Build history of the part. All positions in model axes, mm. Round coordinates to 2 decimals unless told otherwise and drop trailing zeros. Write each loop counter-clockwise with the first axis right and the second up, starting at its lowest first coordinate (ties: lowest second). Pieces come first, ordered by that corner, then holes. Notation, with made-up numbers: (-30.5, 4.25) -> (-8.5, 4.25) arc R17 ccw to (-8.5, 23.25) -> close; hole circle Ø7 at (-34.5, 27.5). An arc over 180 degrees is marked (long way). Answer as CSV lines item,"result".
from build123d import *

# Parameters (mm, degrees)
SKETCH1_R           = 78.359
BOSS_EXTRUDE1_DEPTH = 228.6
SKETCH2_W           = 3.175
SKETCH2_H           = 194.31
CUT_EXTRUDE1_DEPTH  = 203.2
SKETCH5_W           = 194.31
SKETCH5_H           = 3.175
CUT_EXTRUDE2_DEPTH  = 203.2


with BuildPart() as part:
    # Sketch1 → Boss-Extrude1 (new body)
    with BuildSketch(Plane.XY):
        Polygon((76.286003624, -41.721564111), (83.443951376, 24.440749568), (41.721564111, 76.286003624), (-24.440749568, 83.443951376), (-76.286003624, 41.721564111), (-83.443951376, -24.440749568), (-41.721564111, -76.286003624), (24.440749568, -83.443951376), align=None)
        Circle(SKETCH1_R, mode=Mode.SUBTRACT)
    extrude(amount=BOSS_EXTRUDE1_DEPTH)

    # Sketch2 → Cut-Extrude1 (cut)
    with BuildSketch(Plane(origin=(8.640407271, 79.8649775, 0), x_dir=(0.99419859, -0.107560047, 0), z_dir=(0.107560047, 0.99419859, 0))):
        with Locations((0, -122.555)):
            Rectangle(SKETCH2_W, SKETCH2_H)
    extrude(amount=-CUT_EXTRUDE1_DEPTH, mode=Mode.SUBTRACT)

    # Sketch5 → Cut-Extrude2 (cut)
    with BuildSketch(Plane(origin=(-79.8649775, 8.640407271, 0), x_dir=(0, 0, 1), z_dir=(-0.99419859, 0.107560047, 0))):
        with Locations((122.555, 0)):
            Rectangle(SKETCH5_W, SKETCH5_H)
    extrude(amount=-CUT_EXTRUDE2_DEPTH, mode=Mode.SUBTRACT)


solid = part.part
1. Cut at C-C, the plane x = 0. Write the cut outline in (y, z).
Results found:
outline,"(-80.8, 0) -> (-78.36, 0) -> (-78.36, 228.6) -> (-80.8, 228.6) -> close; (78.36, 0) -> (80.8, 0) -> (80.8, 228.6) -> (78.36, 228.6) -> close"
2. Cut at B-B, the plane y = 53. Write the cut outline in (x, z).
Results found:
outline,"(-62.27, 0) -> (-57.72, 0) -> (-57.72, 228.6) -> (-62.27, 228.6) -> close; (57.72, 0) -> (60.46, 0) -> (60.46, 228.6) -> (57.72, 228.6) -> close"
3. Cut at A-A, the plane z = 193. Write the cut outline in (x, y).
Results found:
outline,"(-83.44, -24.44) -> (-41.72, -76.29) -> (-10.22, -79.69) -> (-10, -77.72) arc R78.36 cw to (-78.06, 6.85) -> (-80.04, 7.06) -> close; (-79.69, 10.22) -> (-77.72, 10) arc R78.36 cw to (6.85, 78.06) -> (7.06, 80.04) -> (-24.44, 83.44) -> (-76.29, 41.72) -> close; (-7.06, -80.04) -> (24.44, -83.44) -> (76.29, -41.72) -> (79.69, -10.22) -> (77.72, -10) arc R78.36 cw to (-6.85, -78.06) -> close; (10, 77.72) arc R78.36 cw to (78.06, -6.85) -> (80.04, -7.06) -> (83.44, 24.44) -> (41.72, 76.29) -> (10.22, 79.69) -> close"
4. Mould opens along X. For faces 1 (the flat face through (-79.02, 16.45, 112.7)), 2 (the cylindrical face through (74.74, 23.54, 112.7)), 3 (the flat face through (-75, 25, 0)) say: +X half, -X half, draft (parallel to the pull), parting line (faces both ways), or undercut.
Results found:
face 1,"-X half"
face 2,"undercut"
face 3,"draft"
5. Drop flat-ended pins along their axis: pin 1 Ø6 at (y, z) = (61, 29.5) entering from +X; pin 2 Ø12 at (x, z) = (58, 50) entering from -Y; pin 3 Ø12 at (y, z) = (-1, 191) entering from +X; pin 4 Ø0.7 at (x, y) = (-9, -79) entering from -Z. Give the stop position or say it passes through.
Results found:
pin 1,"stops at x = 56.44"
pin 2,"stops at y = -61.27"
pin 3,"stops at x = 81.34"
pin 4,"stops at z = 0"
6. Probe line 1 along X through (y, z) = (-69, 126.5); line 2 along Y through (x, z) = (0, 105.5); line 3 along Y through (x, z) = (-57.5, 30). List the from-to ranges inside material, lowest first.
Results found:
line 1,"x = -47.58 to -37.14, 37.14 to 42.39"
line 2,"y = -80.8 to -78.36, 78.36 to 80.8"
line 3,"y = -56.68 to -53.23, 53.23 to 56.84"
